```python
from build123d import *

# Parameters (mm, degrees)
F1_DEPTH = 76.2
F3_DEPTH = 19.05


with BuildPart() as f1:
    # F0 (on Top) → F1 (new body)
    with BuildSketch(Plane.XY):
        with BuildLine():
            ThreePointArc((19.05, 12.7), (17.190128, 17.190128), (12.7, 19.05))
            Line((12.7, 19.05), (-12.7, 19.05))
            ThreePointArc((-12.7, 19.05), (-17.190128, 17.190128), (-19.05, 12.7))
            Line((-19.05, 12.7), (-19.05, -12.7))
            ThreePointArc((-19.05, -12.7), (-17.190128, -17.190128), (-12.7, -19.05))
            Line((-12.7, -19.05), (12.7, -19.05))
            ThreePointArc((12.7, -19.05), (17.190128, -17.190128), (19.05, -12.7))
            Line((19.05, -12.7), (19.05, 12.7))
        make_face()
    extrude(amount=F1_DEPTH)

    # F2 (on Front) → F3 (cut, symmetric)
    with BuildSketch(Plane.XZ):
        Polygon((18.924247, 0), (-19.05, 21.924442), (-19.05, 0), align=None)
    extrude(amount=F3_DEPTH, both=True, mode=Mode.SUBTRACT)


solid = f1.part
```
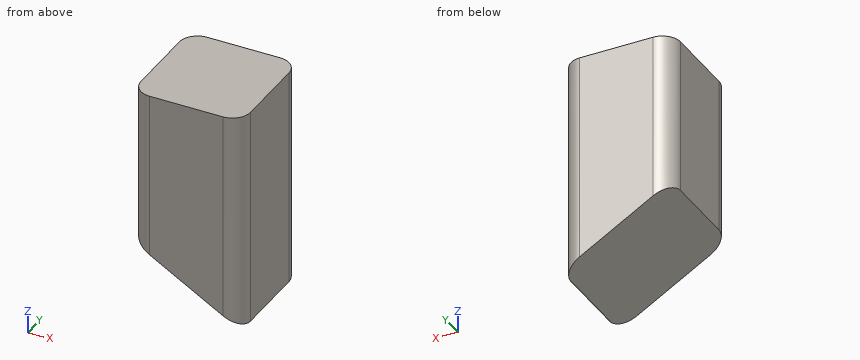
Check sheet for the modelled part. Datum: model origin and axes. Units: mm. Round coordinates to 2 decimals unless told otherwise and drop trailing zeros. Order: outer loops, then holes, each group sorted by start corner. A loop starts at its lowest first (then second) coordinate and runs counter-clockwise, first axis right, second up. Notation, with made-up numbers: (-2, 47.25) - (24, 47.25) arc R14 cw to (24, 74.25) - close; hole circle Ø5 at (51.25, 69). An arc over 180 degrees is marked (long way). Answer as CSV lines item,"result". Start each with the question number.
1) Section check A-A (z = 49.5). Record the cut outline in (x, y).
2) Scan lines: probe 1 along Y at (x, z) = (13, 31.5); probe 2 along Z at (x, y) = (6.5, -12); probe 3 along X at (y, z) = (17, 23.5). Record each from-to range of solid material in increasing order.
3) Section check C-C (x = 9.5). Record the cut outline in (y, z), then the cut area to 3 significant figures.
4) Section check D-D (x = -15). Record the cut outline in (y, z), then the cut area to 3 significant figures.
5) Section check B-B (y = 2). Record the cut outline in (x, z).
6) Depth check by flat-ended pin: pin 1 (1.5 mm diameter, centred on x = -9.5, z = 13.5, fed in from -Y); pin 2 (3 mm diameter, centred on x = -7, y = -14.5, fed in from -Z); pin 3 (3 mm diameter, centred on y = -12, z = 14.5, fed in from -X); pin 4 (6 mm diameter, centred on x = -4, y = -1, fed in from -Z). Enter the tip coordinate at first touch or a pass-through.
Determined:
1,outline,"(-19.05, -12.7) arc R6.35 ccw to (-12.7, -19.05) - (12.7, -19.05) arc R6.35 ccw to (19.05, -12.7) - (19.05, 12.7) arc R6.35 ccw to (12.7, 19.05) - (-12.7, 19.05) arc R6.35 ccw to (-19.05, 12.7) - close"
2,probe 1,"-19.04 to 19.04"
2,probe 2,"7.17 to 76.2"
2,probe 3,"-17.37 to 17.37"
3,outline,"(-19.05, 5.44) - (19.05, 5.44) - (19.05, 76.2) - (-19.05, 76.2) - close"
3,area,"2,700 mm^2"
4,outline,"(-18.62, 19.59) - (18.62, 19.59) - (18.62, 76.2) - (-18.62, 76.2) - close"
4,area,"2,110 mm^2"
5,outline,"(-19.05, 21.92) - (18.92, 0) - (19.05, 0) - (19.05, 76.2) - (-19.05, 76.2) - close"
6,pin 1,"through"
6,pin 2,"z = 14.1"
6,pin 3,"x = -8.79"
6,pin 4,"z = 11.5"
